Verification items for the finished model (mm, model axes). Round coordinates to 2 decimals unless told otherwise and drop trailing zeros. Write each loop counter-clockwise with the first axis right and the second up, starting at its lowest first coordinate (ties: lowest second). Pieces come first, ordered by that corner, then holes. Notation, with made-up numbers: M -14.75,50 L 12.25,50 A24 cw 12.25,81 Z; hole C -31,54.25 d11. An arc over 180 degrees is marked long. One line per item, written item: value. Start each with the question number.
Item 1: Section check C-C, the plane z = 5.25. State how many separate pieces and enclosed holes the cut face has, then the cut area to 3 significant figures.
Item 2: Section check A-A, the plane y = -105. Record the cut outline in (x, z).
Item 3: Thickness scan on probe 1 along X at (y, z) = (33, -6.25); probe 2 along Y at (x, z) = (124.5, -1). Record the ranges inside material, lowest first. Write a range as from..to.
from build123d import *

# Parameters (mm, degrees)
SKETCH1_W           = 145
SKETCH1_H           = 145
BOSS_EXTRUDE2_DEPTH = 7.5
SKETCH3_W           = 145
SKETCH3_H           = 145
SKETCH3_W_2         = 115
SKETCH3_H_2         = 115
BOSS_EXTRUDE4_DEPTH = 12
SKETCH4_R           = 0.275
CUT_EXTRUDE1_DEPTH  = 224.243140992
SKETCH5_R           = 2
CUT_EXTRUDE2_DEPTH  = 224.243140992
FILLET1_R           = 4


with BuildPart() as part:
    # Sketch1 → Boss-Extrude2 (new, symmetric)
    with BuildSketch(Plane.XY):
        Polygon((-157.5, 157.5), (157.5, 157.5), (157.5, -157.5), (-157.5, -157.5), (-157.5, -2.5), (-157.5, 2.5), align=None)
        with Locations((-75, 75)):
            Rectangle(SKETCH1_W, SKETCH1_H, mode=Mode.SUBTRACT)
        with Locations((-75, -75)):
            Rectangle(SKETCH1_W, SKETCH1_H, mode=Mode.SUBTRACT)
        with Locations((75, 75)):
            Rectangle(SKETCH1_W, SKETCH1_H, mode=Mode.SUBTRACT)
        with Locations((75, -75)):
            Rectangle(SKETCH1_W, SKETCH1_H, mode=Mode.SUBTRACT)
    extrude(amount=BOSS_EXTRUDE2_DEPTH, both=True)

    # Sketch3 → Boss-Extrude4 (add)
    # profile 1 of 4: a face of its own
    with BuildSketch(Plane.XY.offset(7.5)):
        with Locations((-75, -75)):
            Rectangle(SKETCH3_W, SKETCH3_H)
        with Locations((-75, -75)):
            Rectangle(SKETCH3_W_2, SKETCH3_H_2, mode=Mode.SUBTRACT)
    # profile 2 of 4: a face of its own
    with BuildSketch(Plane.XY.offset(7.5)):
        with Locations((75, -75)):
            Rectangle(SKETCH3_W, SKETCH3_H)
        with Locations((75, -75)):
            Rectangle(SKETCH3_W_2, SKETCH3_H_2, mode=Mode.SUBTRACT)
    # profile 3 of 4: a face of its own
    with BuildSketch(Plane.XY.offset(7.5)):
        with Locations((75, 75)):
            Rectangle(SKETCH3_W, SKETCH3_H)
        with Locations((75, 75)):
            Rectangle(SKETCH3_W_2, SKETCH3_H_2, mode=Mode.SUBTRACT)
    # profile 4 of 4: a face of its own
    with BuildSketch(Plane.XY.offset(7.5)):
        with Locations((-75, 75)):
            Rectangle(SKETCH3_W, SKETCH3_H)
        with Locations((-75, 75)):
            Rectangle(SKETCH3_W_2, SKETCH3_H_2, mode=Mode.SUBTRACT)
    extrude(amount=-BOSS_EXTRUDE4_DEPTH)

    # Sketch4 → Cut-Extrude1 (cut, through all)
    with BuildSketch(Plane(origin=(0, 0, -7.5), x_dir=(-1, 0, 0), z_dir=(0, 0, -1))):
        with Locations((-1.7, 152.5)):
            Circle(SKETCH4_R)
        with Locations((1.7, 152.5)):
            Circle(SKETCH4_R)
        with Locations((-1.7, 0)):
            Circle(SKETCH4_R)
        with Locations((1.7, 0)):
            Circle(SKETCH4_R)
        with Locations((-152.5, 1.7)):
            Circle(SKETCH4_R)
        with Locations((-152.5, -1.7)):
            Circle(SKETCH4_R)
        with Locations(Location((1.7, -152.5, 0), (0, 0, 180))):
            Circle(SKETCH4_R)
        with Locations(Location((-1.7, -152.5, 0), (0, 0, 180))):
            Circle(SKETCH4_R)
        with Locations(Location((152.5, -1.7, 0), (0, 0, 180))):
            Circle(SKETCH4_R)
        with Locations(Location((152.5, 1.7, 0), (0, 0, 180))):
            Circle(SKETCH4_R)
    extrude(amount=-CUT_EXTRUDE1_DEPTH, mode=Mode.SUBTRACT)

    # Sketch5 → Cut-Extrude2 (cut, through all)
    with BuildSketch(Plane.XY.offset(7.5)):
        with Locations((-27.6, -8)):
            Circle(SKETCH5_R)
        with Locations((-27.6, 8)):
            Circle(SKETCH5_R)
        with Locations((27.6, 8)):
            Circle(SKETCH5_R)
        with Locations((27.6, -8)):
            Circle(SKETCH5_R)
    extrude(amount=-CUT_EXTRUDE2_DEPTH, mode=Mode.SUBTRACT)

    # Fillet1
    fillet1_edges = [part.edges().sort_by_distance(p)[0] for p in [
        (-157.5, 157.5, 0),
        (157.5, 157.5, 0),
        (157.5, -157.5, 0),
        (-157.5, -157.5, 0),
    ]]
    fillet(fillet1_edges, radius=FILLET1_R)


solid = part.part
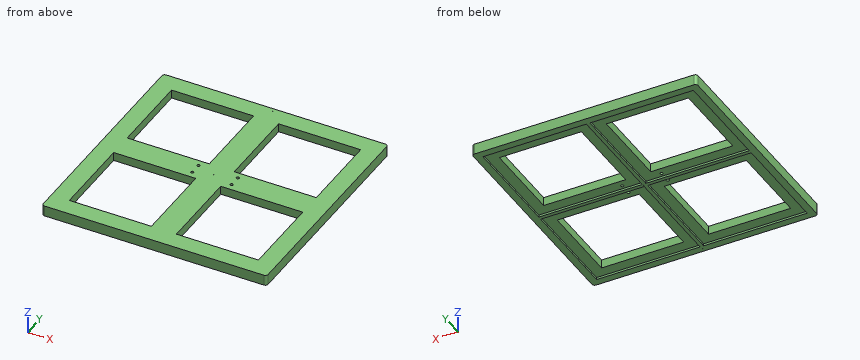
Response values:
1. separate pieces: 1
1. enclosed holes: 18
1. area: 46,300 mm2
2. outline: M -157.5,-7.5 L -147.5,-7.5 L -147.5,-4.5 L -132.5,-4.5 L -132.5,7.5 L -157.5,7.5 Z; M -17.5,-4.5 L -2.5,-4.5 L -2.5,-7.5 L 2.5,-7.5 L 2.5,-4.5 L 17.5,-4.5 L 17.5,7.5 L -17.5,7.5 Z; M 132.5,-4.5 L 147.5,-4.5 L 147.5,-7.5 L 157.5,-7.5 L 157.5,7.5 L 132.5,7.5 Z
3. probe 1: x = -157.5..-147.5, -2.5..2.5, 147.5..157.5
3. probe 2: y = -157.5..-132.5, -17.5..17.5, 132.5..157.5
